Work out the finished part from the listing and answer in its coordinate system (mm). A direction names the side the tool comes from. Round coordinates to 2 decimals unless told otherwise and drop trailing zeros. Order: outer loops, then holes, each group sorted by start corner. A loop starts at its lowest first (then second) coordinate and runs counter-clockwise, first axis right, second up. Notation, with made-up numbers: (62.5, 35.5) - (82.5, 35.5) arc R24 ccw to (82.5, 65.5) - close; hole circle Ø1 at (32, 67). An arc over 180 degrees is marked (long way). Use one line per item in the form item = value. Start each with the question number.
Q1. The part is cut by section A-A on x = 23.75. Determine the outline of the cut face in (y, z), plus the area to 3 significant figures.
Q2. Which of the six approach directions +Z, -Z, +X, -X, +Y, -Y give full straight-line access (tool end or side, diameter ignored) to faces 5 (the flat face through (-1, 7, 0)), 6 (the flat face through (-1, -7, 0)), 7 (the flat face through (1, 10, 1))?
Q3. Find the intervals of material crossed by line 1 (Y direction, x = -23.75, z = 0.2); line 2 (Y direction, x = -45, z = 0.7); line 3 (Z direction, x = 15.5, y = 9), in increasing order. Write a range as [from, to].
Q4. The part is cut by section B-B on z = 0.75. Determine the outline of the cut face in (x, y), plus the area to 3 significant figures.
Q5. Given P1, Ø3, axis at x = -2, y = 6.5, coming from the -Z side, flat-ended and moving along its own axis, determine where the tip first touches the part or whether it passes through.
Q6. The part is cut by section D-D on y = -8.25. Determine the outline of the cut face in (x, z).
Q7. The part is cut by section C-C on y = 0. Determine the outline of the cut face in (x, z).
Q8. For a pull along X with two mould halves and no side action, classify faces 1 (the cylindrical face through (47.575, 0.811, 0.225)), 2 (the flat face through (-50, 0, 1)), 3 (the cylindrical face through (-22.224, 0.481, 0.225)), 4 (the flat face through (-1, 0, -1.6)) as +X half, -X half, draft (parallel to the pull), parting line (faces both ways), or undercut.
from build123d import *

# Parameters (mm, degrees)
F1_DEPTH = 2
F3_DEPTH = 100
F4_R     = 2.7
F4_R_2   = 1.6
F5_DEPTH = 3.601
F6_SIZE  = 1.6


with BuildPart() as f1:
    # F0 (on Top) → F1 (new body)
    with BuildSketch(Plane.XY):
        with BuildLine():
            ThreePointArc((50, 5), (48.535534, 8.535534), (45, 10))
            Line((45, 10), (-45, 10))
            ThreePointArc((-45, 10), (-48.535534, 8.535534), (-50, 5))
            Line((-50, 5), (-50, -5))
            ThreePointArc((-50, -5), (-48.535534, -8.535534), (-45, -10))
            Line((-45, -10), (45, -10))
            ThreePointArc((45, -10), (48.535534, -8.535534), (50, -5))
            Line((50, -5), (50, 5))
        make_face()
    extrude(amount=F1_DEPTH)

    # F2 (on face) → F3 (join, through all)
    with BuildSketch(Plane(origin=(-50, 0, 0), x_dir=(0, -1, 0), z_dir=(-1, 0, 0))):
        Polygon((-4.5, 0), (-2.9, -1.6), (2.9, -1.6), (4.5, 0), align=None)
    extrude(amount=-F3_DEPTH)

    # F4 (on face) → F5 (cut, through all)
    with BuildSketch(Plane.XY.offset(2)):
        with Locations((-45, 0)):
            Circle(F4_R)
        with Locations((45, 0)):
            Circle(F4_R)
        with Locations((23.75, 0)):
            Circle(F4_R_2)
        with Locations((-23.75, 0)):
            Circle(F4_R_2)
    extrude(amount=-F5_DEPTH, mode=Mode.SUBTRACT)

    # F6
    f6_edges = [f1.edges().sort_by_distance(p)[0] for p in [
        (-50, 0, -1.6),
        (50, 0, -1.6),
    ]]
    chamfer(f6_edges, length=F6_SIZE)


solid = f1.part
Found:
q1.outline = (-10, 0) - (-4.5, 0) - (-2.9, -1.6) - (-1.6, -1.6) - (-1.6, 2) - (-10, 2) - close; (1.6, -1.6) - (2.9, -1.6) - (4.5, 0) - (10, 0) - (10, 2) - (1.6, 2) - close
q1.area = 40.3 mm²
q2.face_5 = -Z, +X, -X, +Y
q2.face_6 = -Z, +X, -X, -Y
q2.face_7 = +Z, -Z, +X, -X, +Y
q3.line_1 = [-10, -1.6], [1.6, 10]
q3.line_2 = [-10, -2.7], [2.7, 10]
q3.line_3 = [0, 2]
q4.outline = (-50, -5) arc R5 ccw to (-45, -10) - (45, -10) arc R5 ccw to (50, -5) - (50, 5) arc R5 ccw to (45, 10) - (-45, 10) arc R5 ccw to (-50, 5) - close; hole circle Ø5.4 at (-45, 0); hole circle Ø3.2 at (-23.75, 0); hole circle Ø3.2 at (23.75, 0); hole circle Ø5.4 at (45, 0)
q4.area = 1,920 mm²
q5.P1 = 0
q6.outline = (-48.8, 0) - (48.8, 0) - (48.8, 2) - (-48.8, 2) - close
q7.outline = (-50, 0) - (-48.4, -1.6) - (-47.7, -1.6) - (-47.7, 2) - (-50, 2) - close; (-42.3, -1.6) - (-25.35, -1.6) - (-25.35, 2) - (-42.3, 2) - close; (-22.15, -1.6) - (22.15, -1.6) - (22.15, 2) - (-22.15, 2) - close; (25.35, -1.6) - (42.3, -1.6) - (42.3, 2) - (25.35, 2) - close; (47.7, -1.6) - (48.4, -1.6) - (50, 0) - (50, 2) - (47.7, 2) - close
q8.face_1 = undercut
q8.face_2 = -X half
q8.face_3 = undercut
q8.face_4 = draft
